Study the drawing (mm; zero at the part's minimum x, y, z) and answer. Give positions to 0.01 mm unless a question says otherwise; leave off trailing zeros. Order: outer loops, then holes, each group sorted by start corner. A loop starts at its lowest first (then second) coordinate and runs counter-clockwise, first axis right, second up.
Item 1: Given pin 1 Ø2.5 at (x, z) = (11.95, 17.5) entering from -Y, flat-ended and moving along its own axis, determine where the tip first touches the part or whether it passes through.
Item 2: A cutting plane is placed at A-A (z = 17.5). Write down the section's boundary in (x, y), plus the area to 4 significant figures.
Item 3: Find the intervals of material crossed by line 1 along X through (y, z) = (2.1, 17.5); line 2 along Z through (x, y) = (11, 2.95), in increasing order.
Item 4: A cutting plane is placed at B-B (x = 27.95). Write down the section's boundary in (y, z).
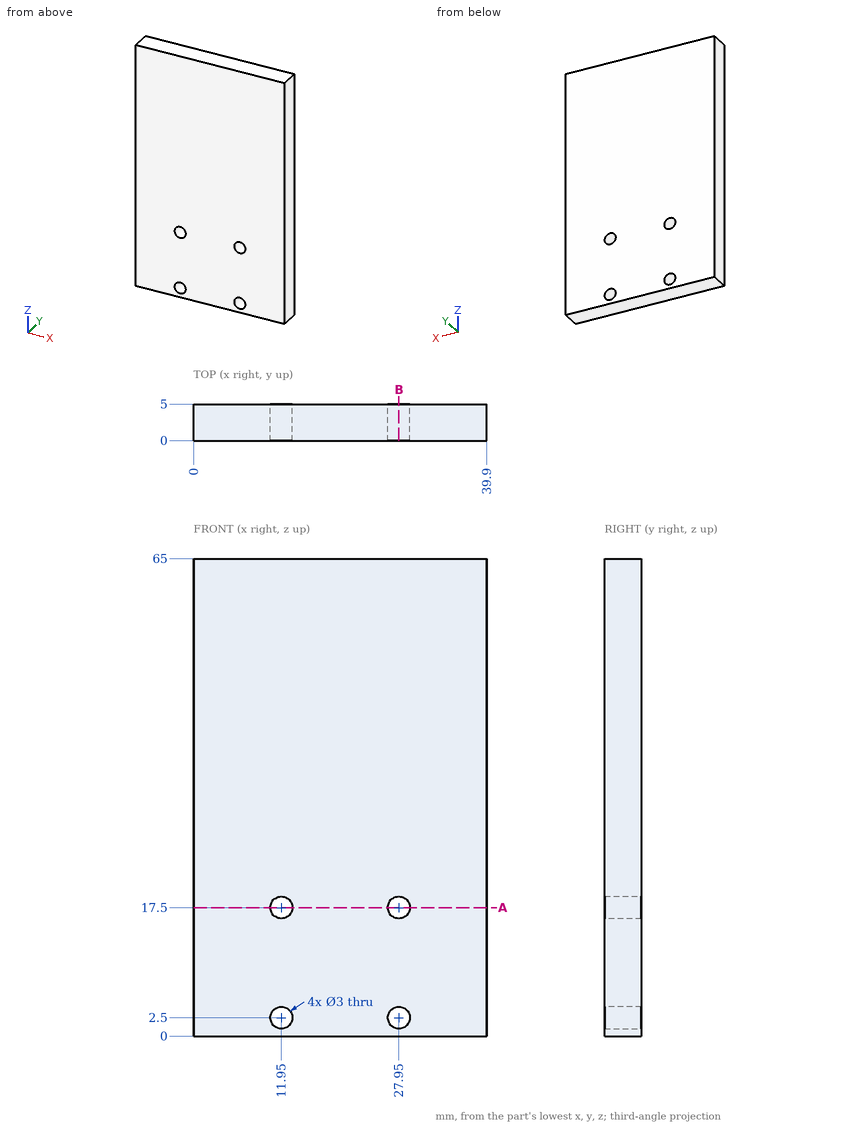
Response values:
1. pin 1: passes through
2. outline: (0, 0) - (10.45, 0) - (10.45, 5) - (0, 5) - close; (13.45, 0) - (26.45, 0) - (26.45, 5) - (13.45, 5) - close; (29.45, 0) - (39.9, 0) - (39.9, 5) - (29.45, 5) - close
2. area: 169.5 mm2
3. line 1: x = 0 to 10.45, 13.45 to 26.45, 29.45 to 39.9
3. line 2: z = 0 to 1.34, 3.66 to 16.34, 18.66 to 65
4. outline: (0, 0) - (5, 0) - (5, 1) - (0, 1) - close; (0, 4) - (5, 4) - (5, 16) - (0, 16) - close; (0, 19) - (5, 19) - (5, 65) - (0, 65) - close
